Source: CAD feature listing. Evaluate the final solid. Frame: model axes, mm. Coordinates: 2 decimals unless noted, no trailing zeros. Order: outer loops, then holes, each group sorted by start corner. A loop starts at its lowest first (then second) coordinate and runs counter-clockwise, first axis right, second up.
Autodesk Inventor part; units mm, degrees
ref_plane "YZ Plane" through (0, 0, 0) normal (1, 0, 0) x (0, 1, 0)
ref_plane "XZ Plane" through (0, 0, 0) normal (0, 1, 0) x (-1, 0, 0)
ref_plane "XY Plane" through (0, 0, 0) normal (0, 0, 1) x (1, 0, 0)
sketch "Skizze1" plane through (0, 0, 0) normal (0, 0, 1) x (1, 0, 0)
  line L0 (-17.5, -6) -> (17.5, -6)
  line L1 (17.5, -6) -> (17.5, 6)
  line L2 (17.5, 6) -> (-17.5, 6)
  line L3 (-17.5, 6) -> (-17.5, -6)
  line L4 (-17.5, -6) -> (17.5, 6) construction
  line L5 (17.5, -6) -> (-17.5, 6) construction
  point P0 (0, 0)
  dimension "d0" = 35
  dimension "d1" = 12
extrude "Extrusion1" add sketch "Skizze1" along normal blind 1.5
sketch "Skizze2" plane through (0, 0, 1.5) normal (0, 0, 1) x (1, 0, 0)
  circle A0 centre (0, 0) radius 2.65
  dimension "d4" = 5.3
extrude "Extrusion2" cut sketch "Skizze2" against normal blind 1.5
sketch "Skizze3" plane through (0, 0, 1.5) normal (0, 0, 1) x (1, 0, 0)
  circle A0 centre (0, 0) radius 3.95
  circle A1 centre (0, 0) radius 2.65
  dimension "d7" = 7.9
extrude "Extrusion3" add sketch "Skizze3" along normal blind 3.5
fillet "Rundung1" radius 0.5 1 edges at (-3.95, 0, 1.5)
equation "\"G_L\" = 0"
equation "\"G_H\" = 0"
equation "\"G_B\" = 0"
properties part number "propstop" material "GEDA Stahl"
1. Section query A-A on x = 0. Return loops of the section in (y, z), plus the area to 3 significant figures.
Findings:
outline: (-6, 0) - (-2.65, 0) - (-2.65, 5) - (-3.95, 5) - (-3.95, 2) arc R0.5 cw to (-4.45, 1.5) - (-6, 1.5) - close; (2.65, 0) - (6, 0) - (6, 1.5) - (4.45, 1.5) arc R0.5 cw to (3.95, 2) - (3.95, 5) - (2.65, 5) - close
area: 19.3 mm2
2. Pin query (flat end, axial travel): P1, Ø1, axis at x = -6.5, y = 4, coming from the +Z side; P2, Ø1.5, axis at x = -12, z = 3, coming from the -Y side. Return the tip coordinate at first contact, or that it passes through.
Findings:
P1: stops at z = 1.5
P2: passes through
3. Draft query along X for faces 1 (the face through (2.45, 1.01, 2.46)), 2 (the face through (17.5, 0, 1)), 3 (the face through (-3.135, 2.404, 3.479)), 4 (the face through (0, -6, 1)). Return one class per face: released by +X, released by -X, zero draft, split by the parting line, or undercut.
Findings:
face 1: undercut
face 2: released by +X
face 3: split by the parting line
face 4: zero draft
4. Section query B-B on y = 0. Return loops of the section in (x, z), plus the area to 3 significant figures.
Findings:
outline: (-17.5, 0) - (-2.65, 0) - (-2.65, 5) - (-3.95, 5) - (-3.95, 2) arc R0.5 cw to (-4.45, 1.5) - (-17.5, 1.5) - close; (2.65, 0) - (17.5, 0) - (17.5, 1.5) - (4.45, 1.5) arc R0.5 cw to (3.95, 2) - (3.95, 5) - (2.65, 5) - close
area: 53.8 mm2
5. Section query C-C on z = 2.65. Return loops of the section in (x, y).
Findings:
outline: circle Ø7.9 at (0, 0); hole circle Ø5.3 at (0, 0)
6. Ray query, line 1 (Y direction, x = 0, z = 2.45); line 2 (Y direction, x = 0, z = 1.4); line 3 (Z direction, x = 5.5, y = -2.75). Return the intervals inside material, ascending.
Findings:
line 1: y = -3.95 to -2.65, 2.65 to 3.95
line 2: y = -6 to -2.65, 2.65 to 6
line 3: z = 0 to 1.5
7. Section query D-D on x = -10. Return loops of the section in (y, z).
Findings:
outline: (-6, 0) - (6, 0) - (6, 1.5) - (-6, 1.5) - close
